Autodesk Inventor part; units mm, degrees
ref_plane "YZ Plane" through (0, 0, 0) normal (1, 0, 0) x (0, 1, 0)
ref_plane "XZ Plane" through (0, 0, 0) normal (0, 1, 0) x (-1, 0, 0)
ref_plane "XY Plane" through (0, 0, 0) normal (0, 0, 1) x (1, 0, 0)
sketch "Sketch1" plane through (0, 0, 0) normal (0, 0, 1) x (1, 0, 0)
  circle A0 centre (0, 0) radius 10
  dimension "d0" = 20
extrude "Extrusion1" add sketch "Sketch1" along normal blind 55
sketch "Sketch2" plane through (0, 0, 55) normal (0, 0, 1) x (1, 0, 0)
  circle A0 centre (0, 0) radius 16
  dimension "d3" = 32
extrude "Extrusion2" add sketch "Sketch2" along normal blind 40
sketch "Sketch3" plane through (0, 0, 0) normal (1, 0, 0) x (0, 1, 0)
  line L0 (16, 55) -> (-16, 55)
  point P0 (0, 0)
  point P1 (0, 81.35)
  dimension "d6" = 26.35
hole "Hole1" at (0, 0, 81.35) direction (-1, 0, 0) diameter 12.7 end through all both
thread "Thread1"
properties part number "CompressionGripAttachment"
For this review, take the finished solid that the model builds, in its own axes (mm). A direction names the side the tool comes from. Round coordinates to 2 decimals unless told otherwise and drop trailing zeros. Order: outer loops, then holes, each group sorted by start corner. A loop starts at its lowest first (then second) coordinate and runs counter-clockwise, first axis right, second up. Notation, with made-up numbers: (38.25, -15.5) -> (90.25, -15.5) arc R28 cw to (90.25, 15.5) -> close; hole circle Ø1 at (-14.5, 24.25). An arc over 180 degrees is marked (long way). Put each result on its own line as item: value.
Q1. Add section A-A on y = 0. Write out the cut boundary in (x, z).
Check result:
outline: (-16, 55) -> (-10, 55) -> (-10, 0) -> (10, 0) -> (10, 55) -> (16, 55) -> (16, 75) -> (-16, 75) -> close; (-16, 87.7) -> (16, 87.7) -> (16, 95) -> (-16, 95) -> close
Q2. Insertion check: pin 1 Ø6 at (x, z) = (-7, 9.5) entering from +Y; pin 2 Ø10 at (y, z) = (-0.5, 31) entering from +X; pin 3 Ø6 at (x, z) = (-11.5, 72) entering from +Y; pin 4 Ø11.5 at (y, z) = (0, 81.35) entering from -X. Each pin has a flat end and moves straight along its axis. Give the tip position at first contact, or say it passes through.
Check result:
pin 1: y = 9.17
pin 2: x = 10
pin 3: y = 13.56
pin 4: through
Q3. Add section D-D on z = 38. Write out the cut boundary in (x, y).
Check result:
outline: circle Ø20 at (0, 0)
Q4. Add section C-C on z = 80.5. Write out the cut boundary in (x, y).
Check result:
outline: (-14.71, -6.29) arc R16 ccw to (14.71, -6.29) -> close; (-14.71, 6.29) -> (14.71, 6.29) arc R16 ccw to start
Q5. For probe 1 along Z at (x, y) = (5, 0); probe 2 along Z at (x, y) = (1.5, 14); probe 3 along Y at (x, z) = (3, 81), list the stretches that pass through material, from the lowest coordinate up. Write a range as [from, to].
Check result:
probe 1: [0, 75], [87.7, 95]
probe 2: [55, 95]
probe 3: [-15.72, -6.34], [6.34, 15.72]
Q6. Add section B-B on x = 0. Write out the cut boundary in (y, z).
Check result:
outline: (-16, 55) -> (-10, 55) -> (-10, 0) -> (10, 0) -> (10, 55) -> (16, 55) -> (16, 95) -> (-16, 95) -> close; hole circle Ø12.7 at (0, 81.35)
Q7. Mouldability with a two-part tool opening along Y and no side actions: class faces 1 (the cylindrical face through (-3.47, 15.62, 74.72)), 2 (the cylindrical face through (-0.224, -0.279, 87.694)), 3 (the flat face through (-0.2, -10.4, 55)) as pulls with the +Y half, pulls with the -Y half, needs draft (parallel to the pull), parting line crosses it, or undercut.
Check result:
face 1: parting line crosses it
face 2: undercut
face 3: needs draft
Q8. Machinability: for faces 4 (the cylindrical face through (-2.17, 9.76, 27.12)), 5 (the flat face through (0, 0, 0)), which of the approach directions +Z, -Z, +X, -X, +Y, -Y give a long, thin tool a straight path to every point of the face, cutting with its end or side? Answer none if there is none.
Check result:
face 4: -Z
face 5: -Z, +X, -X, +Y, -Y
